Design review of the part shown in the three views and the two pictorial views. Dimensions are in mm from the part's minimum x, y and z. A direction names the side the tool comes from. Round coordinates to 2 decimals unless told otherwise and drop trailing zeros. Order: outer loops, then holes, each group sorted by start corner. A loop starts at its lowest first (then second) coordinate and runs counter-clockwise, first axis right, second up.
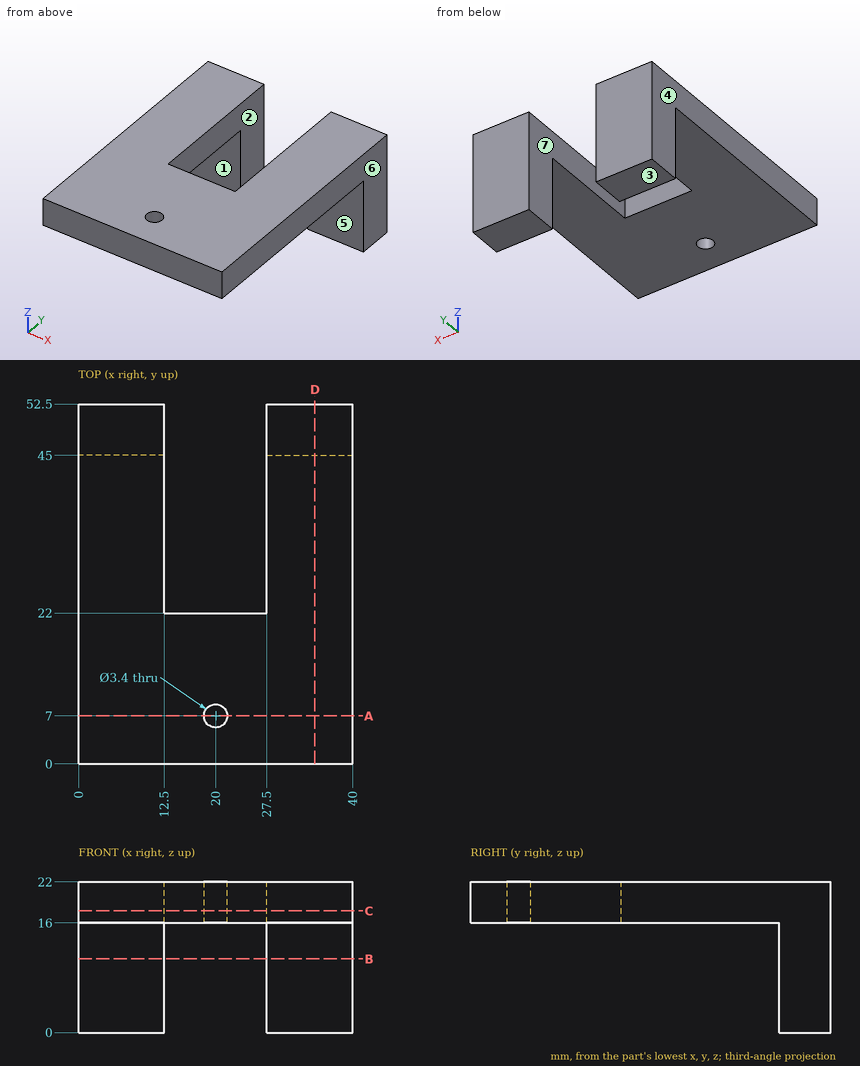
(1) Insertion check: pin 1 (6 mm diameter, centred on x = 5, z = 9.5, fed in from -Y); pin 2 (2 mm diameter, centred on x = 13, y = 21.5, fed in from -Z); pin 3 (6.5 mm diameter, centred on x = 17, z = 18, fed in from +Y). Each pin has a flat end and moves straight along its axis. Give the tip position at first contact, or say it passes through.
Data:
pin 1: stops at y = 45
pin 2: stops at z = 16
pin 3: stops at y = 22
(2) To check wall thickness, follow probe 1 along Y at (x, z) = (20, 19); probe 2 along X at (y, z) = (7, 17.45); probe 3 along X at (y, z) = (46, 7.5). State the ranges of each line that lie inside material, in increasing order.
Data:
probe 1: y = 0 to 5.3, 8.7 to 22
probe 2: x = 0 to 18.3, 21.7 to 40
probe 3: x = 0 to 12.5, 27.5 to 40
(3) Consider section A-A (y = 7). Write out the cut boundary in (x, z), and give its area (3 significant figures).
Data:
outline: (0, 16) - (18.3, 16) - (18.3, 22) - (0, 22) - close; (21.7, 16) - (40, 16) - (40, 22) - (21.7, 22) - close
area: 220 mm2
(4) Consider section B-B (z = 10.75). Write out the cut boundary in (x, y).
Data:
outline: (0, 45) - (12.5, 45) - (12.5, 52.5) - (0, 52.5) - close; (27.5, 45) - (40, 45) - (40, 52.5) - (27.5, 52.5) - close
(5) Draft analysis for pull direction X (two halves, no side actions). For the marked faces 4, 5, 6 and 7, state which applies: pulls with the +X half, pulls with the -X half, needs draft (parallel to the pull), parting line crosses it, or undercut.
Data:
face 4: pulls with the -X half
face 5: needs draft
face 6: pulls with the +X half
face 7: undercut
(6) Consider section C-C (z = 17.75). Write out the cut boundary in (x, y).
Data:
outline: (0, 0) - (40, 0) - (40, 52.5) - (27.5, 52.5) - (27.5, 22) - (12.5, 22) - (12.5, 52.5) - (0, 52.5) - close; hole circle Ø3.4 at (20, 7)
(7) Consider section D-D (x = 34.5). Write out the cut boundary in (y, z).
Data:
outline: (0, 16) - (45, 16) - (45, 0) - (52.5, 0) - (52.5, 22) - (0, 22) - close
(8) For the marked faces 1, 2 and 3, list the 3-axis set-ups (+Z, -Z, +X, -X, +Y, -Y) from which the entire face can be reached by the end or side of a thin tool; tool diameter is ignored.
Data:
face 1: -Z, +X, -X, -Y
face 2: +Z, -Z, +Y
face 3: -Z, +X, -X, +Y, -Y
